The figure shows three views and two pictorial views of one solid part (mm, origin at its lowest corner). Answer the questions. A direction names the side the tool comes from. Give positions to 0.01 mm unless a question says otherwise; leave off trailing zeros. Loops run counter-clockwise (first coordinate to the right, second up) from the corner with the lowest first, then second, coordinate; pieces in that order, holes last. Notation, with made-up numbers: M 84.5,68 L 118.5,68 A15 ccw 118.5,75 Z; hole C -22,18.25 d10. An arc over 180 degrees is marked long. Write item = value, one per line. Start each with the question number.
1. Section D-D on x = 25 is taken. Determine the outline of the cut face in (y, z).
2. Consider L1, parallel to Z at x = 8.5, y = 22; L2, parallel to Y at x = 22.5, z = 3 (1 decimal). Determine where each line is inside the solid, lowest interval first. Write a range as [from, to].
3. Section A-A on z = 30 is taken. Determine the outline of the cut face in (x, y), plus the area to 3 significant figures.
4. For the marked faces 1 and 2, determine the directions among +Z, -Z, +X, -X, +Y, -Y from which every point of the face is accessible in a straight line to the end or side of a thin tool.
5. Flat-ended cylindrical pins translate along their axes: pin 1 Ø6 at (x, y) = (30, 33) entering from +Z; pin 2 Ø1.5 at (x, z) = (13, 37) entering from +Y. Find the tip coordinate at first contact, or state that the pin passes through.
6. Section B-B on x = 20.5 is taken. Determine the outline of the cut face in (y, z), plus the area to 3 significant figures.
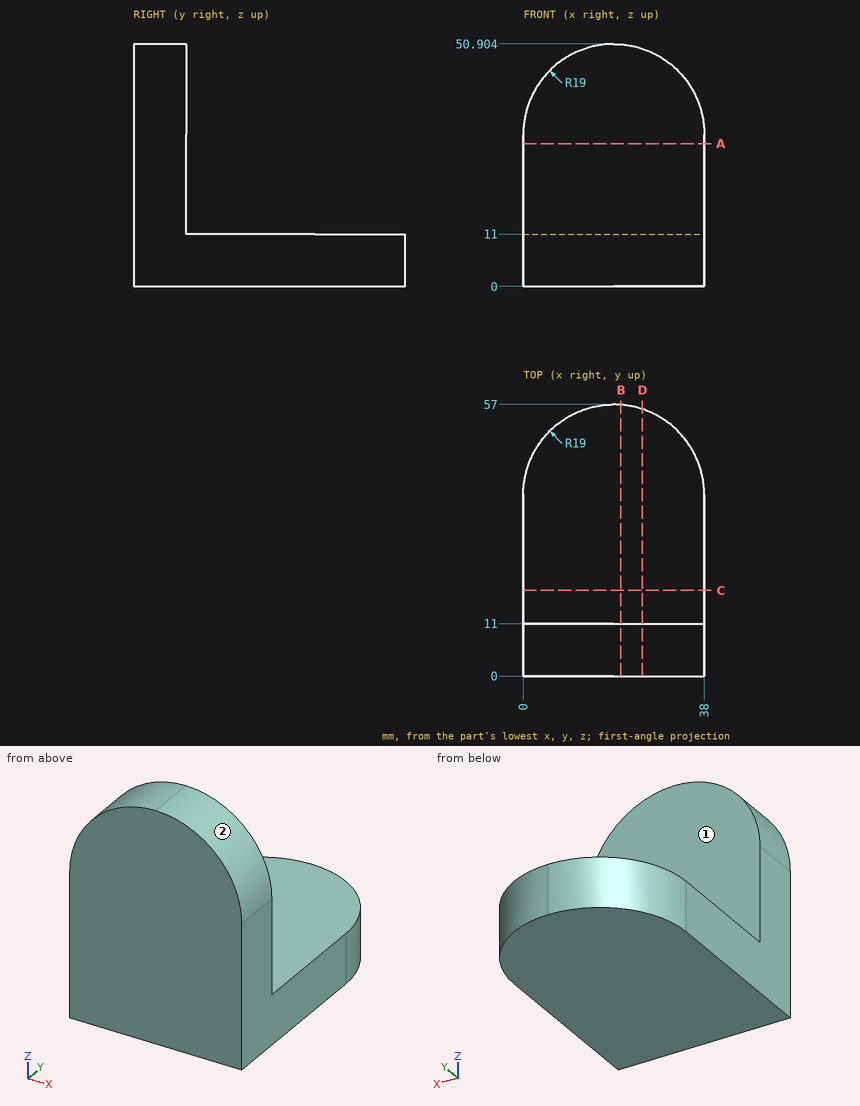
Verdict:
q1.outline = M 0,0 L 56.03,0 L 56.03,11 L 11,11 L 11,49.93 L 0,49.93 Z
q2.L1 = [0, 11]
q2.L2 = [0, 56.7]
q3.outline = M 0,0 L 38,0 L 38,11 L 0,11 Z
q3.area = 418 mm2
q4.face_1 = +Z, +X, -X, +Y
q4.face_2 = +Z, +X, +Y, -Y
q5.pin_1 = 11
q5.pin_2 = 11
q6.outline = M 0,0 L 56.94,0 L 56.94,11 L 11,11 L 11,50.84 L 0,50.84 Z
q6.area = 1,060 mm2
